The model under review builds one solid part; all positions refer to its coordinate system, in mm. A direction names the side the tool comes from. Coordinates: 2 decimals unless noted, no trailing zeros. Order: outer loops, then holes, each group sorted by start corner. A loop starts at its lowest first (then second) coordinate and runs counter-clockwise, first axis right, second up. Notation, with made-up numbers: (49, 83.25) - (63, 83.25) arc R10 ccw to (63, 93.25) - close; hole circle Ø1 at (12, 49.25). An arc over 180 degrees is marked (long way). Answer in a Markdown table with one row per item.
```python
from build123d import *

# Parameters (mm, degrees)
SKETCH_1_W                  = 40
SKETCH_1_H                  = 40
SKETCH_1_W_2                = 30
SKETCH_1_H_2                = 30
EXTRUDE_1_DEPTH             = 1400
HOLE_WIZARD_M41_D           = 3.3
HOLE_WIZARD_M41_DEPTH       = 11.5
HOLE_WIZARD_M41_CSINK_D     = 4.05
HOLE_WIZARD_M41_CSINK_ANGLE = 120
HOLE_WIZARD_M41_TIP         = 0.991420021
HOLE_WIZARD_M42_D           = 3.3
HOLE_WIZARD_M42_DEPTH       = 11.5
HOLE_WIZARD_M42_CSINK_D     = 4.05
HOLE_WIZARD_M42_CSINK_ANGLE = 120
HOLE_WIZARD_M42_TIP         = 0.991420021
HOLE_WIZARD_M43_D           = 3.3
HOLE_WIZARD_M43_DEPTH       = 11.5
HOLE_WIZARD_M43_CSINK_D     = 4.05
HOLE_WIZARD_M43_CSINK_ANGLE = 120
HOLE_WIZARD_M43_TIP         = 0.991420021
HOLE_WIZARD_M44_D           = 3.3
HOLE_WIZARD_M44_DEPTH       = 11.5
HOLE_WIZARD_M44_CSINK_D     = 4.05
HOLE_WIZARD_M44_CSINK_ANGLE = 120
HOLE_WIZARD_M44_TIP         = 0.991420021


with BuildPart() as part:
    # Эскиз1 → Вытянуть-Тонкостенный1 (new body)
    with BuildSketch(Plane.XY):
        with Locations((20, 20)):
            Rectangle(SKETCH_1_W, SKETCH_1_H)
        with Locations((20, 20)):
            Rectangle(SKETCH_1_W_2, SKETCH_1_H_2, mode=Mode.SUBTRACT)
    extrude(amount=EXTRUDE_1_DEPTH)

    # Отверстие обработанное метчиком M41
    with Locations(Plane.ZY):
        with Locations((1030, 30), (1010, 30), (1030, 10), (1010, 10)):
            CounterSinkHole(HOLE_WIZARD_M41_D / 2, HOLE_WIZARD_M41_CSINK_D / 2, depth=HOLE_WIZARD_M41_DEPTH, counter_sink_angle=HOLE_WIZARD_M41_CSINK_ANGLE)
            with Locations((0, 0, -(HOLE_WIZARD_M41_DEPTH + HOLE_WIZARD_M41_TIP / 2))):  # 118° drill point
                Cone(0, HOLE_WIZARD_M41_D / 2, HOLE_WIZARD_M41_TIP, mode=Mode.SUBTRACT)

    # Отверстие обработанное метчиком M42
    with Locations(Plane(origin=(40, 0, 0), x_dir=(0, 0, -1), z_dir=(1, 0, 0))):
        with Locations((-598, 30), (-578, 30), (-598, 10), (-578, 10)):
            CounterSinkHole(HOLE_WIZARD_M42_D / 2, HOLE_WIZARD_M42_CSINK_D / 2, depth=HOLE_WIZARD_M42_DEPTH, counter_sink_angle=HOLE_WIZARD_M42_CSINK_ANGLE)
            with Locations((0, 0, -(HOLE_WIZARD_M42_DEPTH + HOLE_WIZARD_M42_TIP / 2))):  # 118° drill point
                Cone(0, HOLE_WIZARD_M42_D / 2, HOLE_WIZARD_M42_TIP, mode=Mode.SUBTRACT)

    # Отверстие обработанное метчиком M43
    with Locations(Plane.XZ):
        with Locations((30, 1030), (10, 1030), (30, 1010), (10, 1010)):
            CounterSinkHole(HOLE_WIZARD_M43_D / 2, HOLE_WIZARD_M43_CSINK_D / 2, depth=HOLE_WIZARD_M43_DEPTH, counter_sink_angle=HOLE_WIZARD_M43_CSINK_ANGLE)
            with Locations((0, 0, -(HOLE_WIZARD_M43_DEPTH + HOLE_WIZARD_M43_TIP / 2))):  # 118° drill point
                Cone(0, HOLE_WIZARD_M43_D / 2, HOLE_WIZARD_M43_TIP, mode=Mode.SUBTRACT)

    # Отверстие обработанное метчиком M44
    with Locations(Plane(origin=(0, 40, 0), x_dir=(-1, 0, 0), z_dir=(0, 1, 0))):
        with Locations((-6, 550), (-26, 550), (-6, 530), (-26, 530)):
            CounterSinkHole(HOLE_WIZARD_M44_D / 2, HOLE_WIZARD_M44_CSINK_D / 2, depth=HOLE_WIZARD_M44_DEPTH, counter_sink_angle=HOLE_WIZARD_M44_CSINK_ANGLE)
            with Locations((0, 0, -(HOLE_WIZARD_M44_DEPTH + HOLE_WIZARD_M44_TIP / 2))):  # 118° drill point
                Cone(0, HOLE_WIZARD_M44_D / 2, HOLE_WIZARD_M44_TIP, mode=Mode.SUBTRACT)


solid = part.part
```
Item 1: We need section A-A, the plane z = 87.5. Write out the cut boundary in (x, y), then the cut area to 3 significant figures.
Check values:
| item | result |
|---|---|
| outline | (0, 0) - (40, 0) - (40, 40) - (0, 40) - close; hole (5, 5) - (35, 5) - (35, 35) - (5, 35) - close |
| area | 700 mm^2 |
Item 2: Mouldability with a two-part tool opening along Y and no side actions: class faces 3 (the face through (5, 20, 690)), 4 (the face through (20, 5, 690)), 5 (the face through (20, 40, 690)), 6 (the face through (20, 0, 690)) as +Y half, -Y half, draft (parallel to the pull), parting line (faces both ways), or undercut.
Check values:
| item | result |
|---|---|
| face 3 | undercut |
| face 4 | undercut |
| face 5 | +Y half |
| face 6 | -Y half |
Item 3: Tool access review of faces 1 (the face through (35, 20, 690)), 2 (the face through (0, 20, 690)): name each direction out of +Z, -Z, +X, -X, +Y, -Y from which nothing blocks a thin tool from reaching the whole face with its end or side.
Check values:
| item | result |
|---|---|
| face 1 | +Z, -Z |
| face 2 | +Z, -Z, -X, +Y, -Y |
Item 4: Clearance check with flat-ended pins moving along their axes: pin 1 Ø9 at (y, z) = (17.5, 376) entering from -X; pin 2 Ø2.5 at (x, z) = (10, 1030) entering from -Y; pin 3 Ø2 at (y, z) = (30, 1030) entering from -X; pin 4 Ø3 at (y, z) = (30, 598) entering from +X. State where each tip first meets the part, or that it passes through.
Check values:
| item | result |
|---|---|
| pin 1 | x = 0 |
| pin 2 | y = 35 |
| pin 3 | x = 35 |
| pin 4 | x = 5 |
Item 5: To check wall thickness, follow line 1 (Y direction, x = 37.85, z = 598); line 2 (Z direction, x = 30, y = 3); line 3 (Y direction, x = 18.5, z = 250.5). State the ranges of each line that lie inside material, in increasing order. Write a range as from..to.
Check values:
| item | result |
|---|---|
| line 1 | 0..8.35, 11.65..28.35, 31.65..40 |
| line 2 | 0..1008.35, 1011.65..1028.35, 1031.65..1400 |
| line 3 | 0..5, 35..40 |
